from build123d import *

# Parameters (mm, degrees)
BOSS_EXTRUDE1_DEPTH = 50
SKETCH10_R          = 3.425
CUT_EXTRUDE5_DEPTH  = 10
SKETCH11_W          = 80
SKETCH11_H          = 5
BOSS_EXTRUDE3_DEPTH = 50
SKETCH14_R          = 3.15
CUT_EXTRUDE6_DEPTH  = 10
FILLET1_R           = 1


with BuildPart() as part:
    # Sketch2 → Boss-Extrude1 (new body)
    with BuildSketch(Plane.XY):
        Polygon((-40.506485759, 0), (59.130974018, 0), (59.130974018, 175), (71.870010435, 247.246665631), (13.397315769, 249.004598584), (-40.506485759, 205.829132158), align=None)
        Polygon((59.130974018, 232.587704831), (59.8009874, 236.446158122), (42.633663102, 236.446158122), (13.397315769, 236.446158122), (6.25157797, 230.468732297), (-30.869025982, 199.417263157), (-30.869025982, 107.989726368), (-30.869025982, 10), (0, 10), (49.130974018, 10), (49.130974018, 87.5), (49.130974018, 175), align=None, mode=Mode.SUBTRACT)
    extrude(amount=BOSS_EXTRUDE1_DEPTH)

    # Sketch10 → Cut-Extrude5 (cut)
    with BuildSketch(Plane(origin=(0, 10, 0), x_dir=(1, 0, 0), z_dir=(0, 1, 0))):
        with Locations((-5.851287133, -25)):
            Circle(SKETCH10_R)
        with Locations((24.130974018, -25)):
            Circle(SKETCH10_R)
    extrude(amount=-CUT_EXTRUDE5_DEPTH, mode=Mode.SUBTRACT)

    # Sketch11 → Boss-Extrude3 (add)
    with BuildSketch(Plane.XY.offset(50)):
        with Locations((9.130974018, 155.135730726)):
            Rectangle(SKETCH11_W, SKETCH11_H)
        with Locations((9.130974018, 78.651297101)):
            Rectangle(SKETCH11_W, SKETCH11_H)
    extrude(amount=-BOSS_EXTRUDE3_DEPTH)

    # Sketch14 → Cut-Extrude6 (cut)
    with BuildSketch(Plane(origin=(27.42119444, -4.835096423, 0), x_dir=(0, 0, -1), z_dir=(0.984807753, -0.173648178, 0))):
        with Locations((-25, 221.609342659)):
            Circle(SKETCH14_R)
    extrude(amount=-CUT_EXTRUDE6_DEPTH, mode=Mode.SUBTRACT)

    # Fillet1
    fillet1_edges = [part.edges().sort_by_distance(p)[0] for p in [
        (65.903252947, 213.407502367, 28.15),
    ]]
    fillet(fillet1_edges, radius=FILLET1_R)


solid = part.part
Verification items for the finished model (mm, model axes). A direction names the side the tool comes from. Coordinates: 2 decimals unless noted, no trailing zeros. Order: outer loops, then holes, each group sorted by start corner. A loop starts at its lowest first (then second) coordinate and runs counter-clockwise, first axis right, second up.
1. Go/stop test with flat-tipped pins: pin 1 Ø25 at (x, z) = (20, 19.5) entering from -Y; pin 2 Ø3 at (x, z) = (56.5, 16.5) entering from +Y; pin 3 Ø5.5 at (x, z) = (24.13, 25) entering from +Y; pin 4 Ø2 at (x, z) = (48, 29) entering from +Y. Record where each tip stops, or that it passes through.
Results found:
pin 1: stops at y = 0
pin 2: stops at y = 247.75
pin 3: stops at y = 248.76
pin 4: stops at y = 247.99
2. Sectioned sample at B-B, the plane z = 12.5. Record the cut outline in (x, y), and give its area (3 significant figures).
Results found:
outline: (-40.51, 0) - (59.13, 0) - (59.13, 175) - (71.87, 247.25) - (13.4, 249) - (-40.51, 205.83) - close; hole (-30.87, 10) - (49.13, 10) - (49.13, 76.15) - (-30.87, 76.15) - close; hole (-30.87, 81.15) - (49.13, 81.15) - (49.13, 152.64) - (-30.87, 152.64) - close; hole (-30.87, 157.64) - (49.13, 157.64) - (49.13, 175) - (59.8, 236.45) - (13.4, 236.45) - (-30.87, 199.42) - close
area: 7,250 mm2
3. Sectioned sample at A-A, the plane y = 93.5. Record the cut outline in (x, z), and give its area (3 significant figures).
Results found:
outline: (-40.51, 0) - (-30.87, 0) - (-30.87, 50) - (-40.51, 50) - close; (49.13, 0) - (59.13, 0) - (59.13, 50) - (49.13, 50) - close
area: 982 mm2
4. Set-up check for faces 1 (the face through (-40.506, 104, 25)), 2 (the face through (11, 153, 50)), 3 (the face through (59.131, 86, 25)), 4 (the face through (-30.869, 43, 25)), 5 (the face through (21.41, 5.07, 27.08)): record each of +Z, -Z, +X, -X, +Y, -Y from which the full face is reachable in a straight line by a thin tool's end or side.
Results found:
face 1: +Z, -Z, -X, +Y, -Y
face 2: +Z, +X, -X, +Y, -Y
face 3: +Z, -Z, +X, -Y
face 4: +Z, -Z
face 5: -Y
5. Sectioned sample at D-D, the plane x = 9.5. Record the cut outline in (y, z), and give its area (3 significant figures).
Results found:
outline: (0, 0) - (10, 0) - (10, 50) - (0, 50) - close; (76.15, 0) - (81.15, 0) - (81.15, 50) - (76.15, 50) - close; (152.64, 0) - (157.64, 0) - (157.64, 50) - (152.64, 50) - close; (233.19, 0) - (245.88, 0) - (245.88, 50) - (233.19, 50) - close
area: 1,630 mm2
6. Release check for a two-part mould opening along Y. For faces 6 (the face through (11, 153, 0)), 7 (the face through (-30.869, 178, 25)), 8 (the face through (65.41, 210.62, 19.09)) record: +Y half, -Y half, draft (parallel to the pull), parting line (faces both ways), or undercut.
Results found:
face 6: draft
face 7: undercut
face 8: -Y half
7. Scan lines: line 1 (X direction, y = 2.5, z = 25); line 2 (X direction, y = 145.5, z = 4); line 3 (Y direction, x = 35, z = 11). Record each from-to range of solid material in increasing order.
Results found:
line 1: x = -40.51 to -9.28, -2.43 to 20.71, 27.56 to 59.13
line 2: x = -40.51 to -30.87, 49.13 to 59.13
line 3: y = 0 to 10, 76.15 to 81.15, 152.64 to 157.64, 236.45 to 248.36
8. Sectioned sample at C-C, the plane x = 25. Record the cut outline in (y, z), and give its area (3 significant figures).
Results found:
outline: (0, 0) - (10, 0) - (10, 21.69) - (0, 21.69) - close; (0, 28.31) - (10, 28.31) - (10, 50) - (0, 50) - close; (76.15, 0) - (81.15, 0) - (81.15, 50) - (76.15, 50) - close; (152.64, 0) - (157.64, 0) - (157.64, 50) - (152.64, 50) - close; (236.45, 0) - (248.66, 0) - (248.66, 50) - (236.45, 50) - close
area: 1,540 mm2
